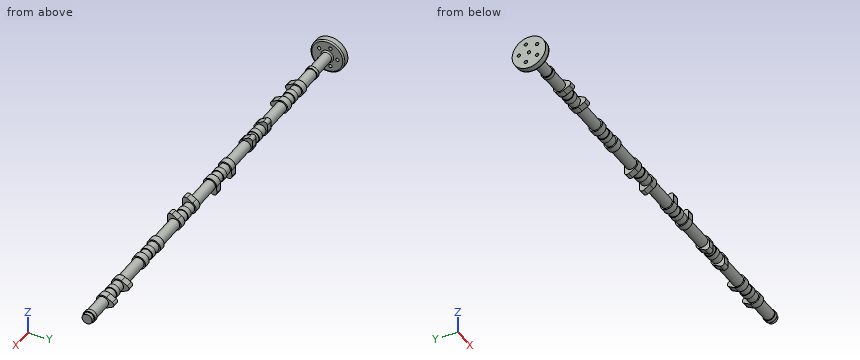
```python
from build123d import *

# Parameters (mm, degrees)
SKETCH1_R             = 8
BOSS_EXTRUDE1_DEPTH   = 47.5
BOSS_EXTRUDE2_START   = 15
BOSS_EXTRUDE2_DEPTH   = 10
SKETCH3_R             = 9
BOSS_EXTRUDE3_DEPTH   = 4
LPATTERN1_COUNT       = 6
LPATTERN1_PITCH       = 95
BODY_MOVE_COPY1_ANGLE = 60
BODY_MOVE_COPY2_ANGLE = 120
BODY_MOVE_COPY3_ANGLE = 60
BODY_MOVE_COPY4_ANGLE = 120
BODY_MOVE_COPY5_ANGLE = 180
BOSS_EXTRUDE4_START   = 10
SKETCH4_R             = 8
BOSS_EXTRUDE4_DEPTH   = 10
BOSS_EXTRUDE5_START   = 5
SKETCH5_R             = 9
BOSS_EXTRUDE5_DEPTH   = 5
SKETCH6_R             = 7.5
BOSS_EXTRUDE6_DEPTH   = 5
SKETCH7_R             = 8
BOSS_EXTRUDE7_DEPTH   = 7.5
SKETCH8_R             = 9
BOSS_EXTRUDE8_DEPTH   = 5
BOSS_EXTRUDE9_START   = 38
SKETCH9_R             = 7.5
BOSS_EXTRUDE9_DEPTH   = 38
SKETCH10_R            = 25
SKETCH10_R_2          = 2.5
BOSS_EXTRUDE10_DEPTH  = 10
FILLET1_R             = 2
SKETCH11_R            = 2.5
CUT_EXTRUDE1_DEPTH    = 10


with BuildPart() as part:
    # Sketch1 → Boss-Extrude1 (new, symmetric)
    with BuildSketch(Plane(origin=(0, 0, 0), x_dir=(0, 0, -1), z_dir=(1, 0, 0))):
        Circle(SKETCH1_R)
    extrude(amount=BOSS_EXTRUDE1_DEPTH, both=True)

    # Sketch2 → Boss-Extrude2 (add)
    with BuildSketch(Plane(origin=(0, 0, 0), x_dir=(0, 0, -1), z_dir=(1, 0, 0)).offset(BOSS_EXTRUDE2_START)):
        with BuildLine():
            Line((-8.746197071, -4.848096202), (-3.807936598, -13.756953924))
            ThreePointArc((-3.807936598, -13.756953924), (0, -16), (3.807936598, -13.756953924))
            Line((3.807936598, -13.756953924), (8.746197071, -4.848096202))
            ThreePointArc((8.746197071, -4.848096202), (0, 10), (-8.746197071, -4.848096202))
        make_face()
    boss_extrude2 = extrude(amount=BOSS_EXTRUDE2_DEPTH)

    # Mirror1: Boss-Extrude2 across plane
    add(boss_extrude2.mirror(Plane(origin=(0, 0, 0), x_dir=(0, 0, 1), z_dir=(1, 0, 0))))

    # Sketch3 → Boss-Extrude3 (add, symmetric)
    with BuildSketch(Plane(origin=(0, 0, 0), x_dir=(0, 0, -1), z_dir=(1, 0, 0))):
        Circle(SKETCH3_R)
    extrude(amount=BOSS_EXTRUDE3_DEPTH, both=True)


with BuildPart() as lpattern1_1:
    # LPattern1: pattern copy
    add(part.part.moved(Location(Vector(1, 0, 0) * (1 * LPATTERN1_PITCH))))


with BuildPart() as lpattern1_2:
    # LPattern1: pattern copy
    add(part.part.moved(Location(Vector(1, 0, 0) * (2 * LPATTERN1_PITCH))))


with BuildPart() as lpattern1_3:
    # LPattern1: pattern copy
    add(part.part.moved(Location(Vector(1, 0, 0) * (3 * LPATTERN1_PITCH))))


with BuildPart() as lpattern1_4:
    # LPattern1: pattern copy
    add(part.part.moved(Location(Vector(1, 0, 0) * (4 * LPATTERN1_PITCH))))


with BuildPart() as lpattern1_5:
    # LPattern1: pattern copy
    add(part.part.moved(Location(Vector(1, 0, 0) * (5 * LPATTERN1_PITCH))))


with BuildPart() as lpattern1_3_1:
    # Body-Move_Copy1: moved
    add(lpattern1_3.part.rotate(Axis((0, 0, 0), (-1, 0, 0)), BODY_MOVE_COPY1_ANGLE))


with BuildPart() as lpattern1_1_1:
    # Body-Move_Copy2: moved
    add(lpattern1_1.part.rotate(Axis((0, 0, 0), (-1, 0, 0)), BODY_MOVE_COPY2_ANGLE))


with BuildPart() as lpattern1_4_1:
    # Body-Move_Copy3: moved
    add(lpattern1_4.part.rotate(Axis((0, 0, 0), (1, 0, 0)), BODY_MOVE_COPY3_ANGLE))


with BuildPart() as lpattern1_2_1:
    # Body-Move_Copy4: moved
    add(lpattern1_2.part.rotate(Axis((0, 0, 0), (1, 0, 0)), BODY_MOVE_COPY4_ANGLE))


with BuildPart() as lpattern1_5_1:
    # Body-Move_Copy5: moved
    add(lpattern1_5.part.rotate(Axis((0, 0, 0), (1, 0, 0)), BODY_MOVE_COPY5_ANGLE))

    # Sketch4 → Boss-Extrude4 (add)
    with BuildSketch(Plane(origin=(522.5, 0, 0), x_dir=(0, 0, -1), z_dir=(1, 0, 0)).offset(BOSS_EXTRUDE4_START)):
        with Locations(Location((0, 0, 0), (0, 0, 180))):
            Circle(SKETCH4_R)
    extrude(amount=-BOSS_EXTRUDE4_DEPTH)

    # Sketch5 → Boss-Extrude5 (add)
    with BuildSketch(Plane(origin=(532.5, 0, 0), x_dir=(0, 0, -1), z_dir=(1, 0, 0)).offset(BOSS_EXTRUDE5_START)):
        with Locations(Location((0, 0, 0), (0, 0, 180))):
            Circle(SKETCH5_R)
    extrude(amount=-BOSS_EXTRUDE5_DEPTH)


with BuildPart() as part_1:
    add(part.part)

    # Combine1: union LPattern1_1, LPattern1_2, LPattern1_3, LPattern1_4, LPattern1_5
    add(lpattern1_1_1.part)
    add(lpattern1_2_1.part)
    add(lpattern1_3_1.part)
    add(lpattern1_4_1.part)
    add(lpattern1_5_1.part)

    # Sketch6 → Boss-Extrude6 (add)
    with BuildSketch(Plane(origin=(537.5, 0, 0), x_dir=(0, 0, -1), z_dir=(1, 0, 0))):
        Circle(SKETCH6_R)
    extrude(amount=BOSS_EXTRUDE6_DEPTH)

    # Sketch7 → Boss-Extrude7 (add)
    with BuildSketch(Plane.ZY.offset(47.5)):
        with Locations(Location((0, 0, 0), (0, 0, 180))):
            Circle(SKETCH7_R)
    extrude(amount=BOSS_EXTRUDE7_DEPTH)

    # Sketch8 → Boss-Extrude8 (add)
    with BuildSketch(Plane.ZY.offset(55)):
        with Locations(Location((0, 0, 0), (0, 0, 180))):
            Circle(SKETCH8_R)
    extrude(amount=BOSS_EXTRUDE8_DEPTH)

    # Sketch9 → Boss-Extrude9 (add)
    with BuildSketch(Plane.ZY.offset(60).offset(BOSS_EXTRUDE9_START)):
        with Locations(Location((0, 0, 0), (0, 0, 180))):
            Circle(SKETCH9_R)
    extrude(amount=-BOSS_EXTRUDE9_DEPTH)

    # Sketch10 → Boss-Extrude10 (add)
    with BuildSketch(Plane.ZY.offset(98)):
        Circle(SKETCH10_R)
        Circle(SKETCH10_R_2, mode=Mode.SUBTRACT)
    extrude(amount=BOSS_EXTRUDE10_DEPTH)

    # Fillet1
    fillet1_edges = [part_1.edges().sort_by_distance(p)[0] for p in [
        (-98, 0, 7.5),
        (-98, 0, -25),
    ]]
    fillet(fillet1_edges, radius=FILLET1_R)

    # Sketch11 → Cut-Extrude1 (cut)
    with BuildSketch(Plane.ZY.offset(108)):
        with Locations((0, 15)):
            Circle(SKETCH11_R)
        with Locations((-14.265847744, 4.635254916)):
            Circle(SKETCH11_R)
        with Locations((-8.816778784, -12.135254916)):
            Circle(SKETCH11_R)
        with Locations((8.816778784, -12.135254916)):
            Circle(SKETCH11_R)
        with Locations((14.265847744, 4.635254916)):
            Circle(SKETCH11_R)
    extrude(amount=-CUT_EXTRUDE1_DEPTH, mode=Mode.SUBTRACT)


solid = part_1.part
```
Verification items for the finished model (mm, model axes). Give positions to 0.01 mm unless a question says otherwise; leave off trailing zeros. Write each loop counter-clockwise with the first axis right and the second up, starting at its lowest first coordinate (ties: lowest second). Pieces come first, ordered by that corner, then holes. Notation, with made-up numbers: (72, 71) - (122, 71) arc R25 ccw to (122, 108) - close; hole circle Ø3 at (49, 16). An arc over 180 degrees is marked (long way). Put each result on its own line as item: value.
Q1. Scan lines: probe 1 along Y at (x, z) = (-105, 0); probe 2 along X at (y, z) = (-6, 12); probe 3 along X at (y, z) = (4, -13.5). Record each from-to range of solid material in increasing order. Write a range as from..to.
Result:
probe 1: -25..-2.5, 2.5..12.5, 17.5..25
probe 2: -108..-98, 260..270, 300..310
probe 3: 165..175, 205..215
Q2. Section check A-A on x = 247. Record the cut outline in (y, z), and give its area (3 significant figures).
Result:
outline: circle Ø16 at (0, 0)
area: 201 mm2
Q3. Depth check by flat-ended pin: P1, Ø8, axis at y = 15, z = 0, coming from the +X side; P2, Ø10, axis at y = 1.5, z = -0.5, coming from the -X side; P3, Ø12, axis at y = 16, z = 17, coming from the +X side; P4, Ø4, axis at x = 51, y = -6, coming from the +Z side. Enter the tip coordinate at first touch or a pass-through.
Result:
P1: x = 500
P2: x = -108
P3: x = -98
P4: z = 6.93
